Here's the drawing with two shaded views (mm, measured from the low corner). I have some questions. A direction names the side the tool comes from. Coordinates: 2 decimals unless noted, no trailing zeros. Write each loop counter-clockwise with the first axis right and the second up, starting at its lowest first coordinate (ties: lowest second). Pieces come first, ordered by that corner, then holes. Notation, with made-up numbers: (14, 50) -> (63, 50) arc R22 cw to (63, 72) -> close; hole circle Ø9 at (82, 64). An arc over 180 degrees is marked (long way). Use one line per item in the form item = value.
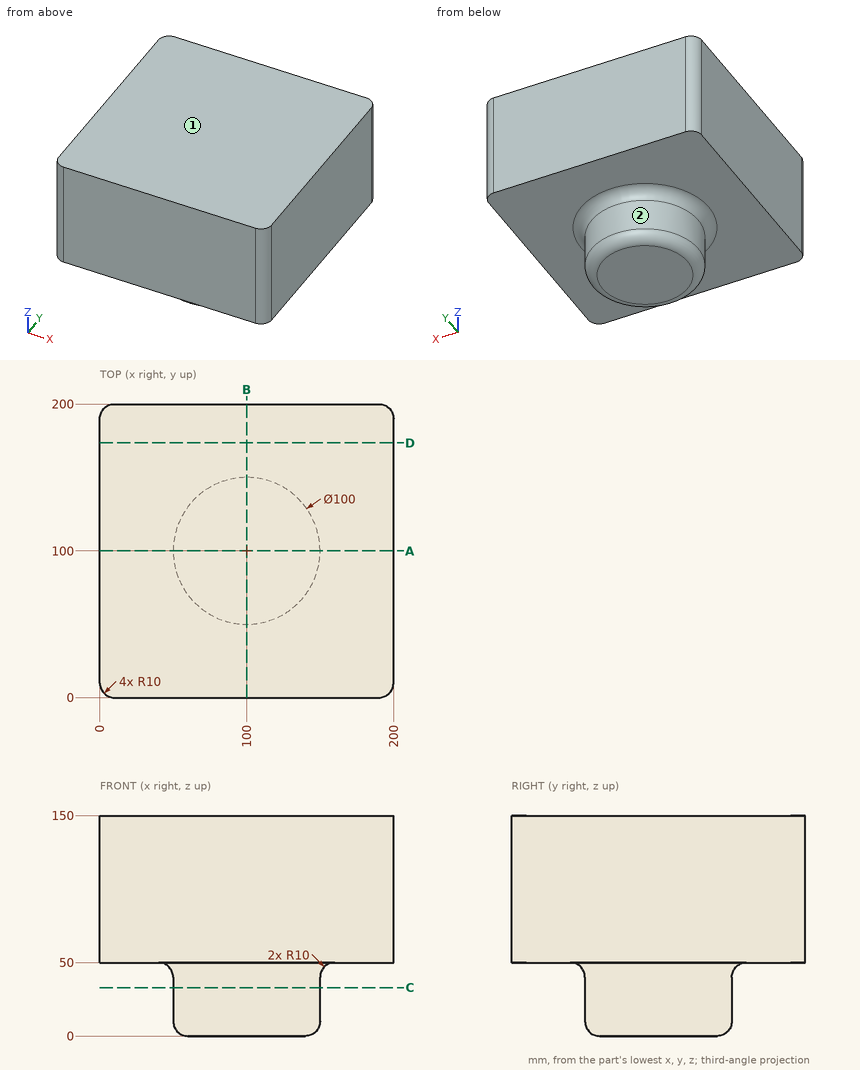
Q1. If I drill on line 1 (Z direction, x = 12.5, y = 142); line 2 (Y direction, x = 192, z = 143); line 3 (X direction, y = 100.5, z = 42), over which ranges is the centre line in solid material (lowest first)? Write a range as from..to.
Return value:
line_1 = 50..150
line_2 = 0.2..199.8
line_3 = 49.8..150.2
Q2. Suppose I cut it at A-A (y = 100). Write out the boundary of the cut face in (x, z).
Return value:
outline = (0, 50) -> (40, 50) arc R10 cw to (50, 40) -> (50, 10) arc R10 ccw to (60, 0) -> (140, 0) arc R10 ccw to (150, 10) -> (150, 40) arc R10 cw to (160, 50) -> (200, 50) -> (200, 150) -> (0, 150) -> close
Q3. For the marked faces 1 and 2, which set-ups out of +Z, -Z, +X, -X, +Y, -Y let a thin tool reach every point of the face, with its end or its side?
Return value:
face_1 = +Z, +X, -X, +Y, -Y
face_2 = -Z
Q4. Suppose I cut it at D-D (y = 173.5). Write out the boundary of the cut face in (x, z), then the cut area to 3 significant figures.
Return value:
outline = (0, 50) -> (200, 50) -> (200, 150) -> (0, 150) -> close
area = 20,000 mm2
Q5. Will these pins go through, and if not, where does the flat tip stop? pin 1 (4 mm diameter, centred on x = 110.5, y = 160.5, fed in from -Z); pin 2 (1.5 mm diameter, centred on y = 94, z = 46, fed in from +X); pin 3 (1 mm diameter, centred on y = 121.5, z = 31, fed in from +X).
Return value:
pin_1 = 49.98
pin_2 = 152.28
pin_3 = 145.38
Q6. Suppose I cut it at C-C (z = 33). Write out the boundary of the cut face in (x, y).
Return value:
outline = circle Ø100 at (100, 100)
